Input: part model. Units: mm. Frame: model coordinates. Coordinates: 2 decimals unless noted, no trailing zeros. Order: outer loops, then holes, each group sorted by start corner. A loop starts at its lowest first (then second) coordinate and runs counter-clockwise, first axis right, second up. Notation, with made-up numbers: (-39.5, 47) -> (9.5, 47) arc R22 ccw to (9.5, 58) -> close; hole circle Ø8 at (11.5, -30.5). An arc over 180 degrees is marked (long way). Use one line per item in the form item = value. Start each with the question number.
1) Pin query (flat end, axial travel): pin 1 (1.5 mm diameter, centred on x = 8, y = 72, fed in from -Z); pin 2 (2 mm diameter, centred on x = 8, y = 112, fed in from +Z); pin 3 (2 mm diameter, centred on x = 8, y = 72, fed in from -Z). Return the tip coordinate at first contact, or that it passes through.
2) Section query B-B on y = 82. Output: boundary loops of the cut face in (x, z).
3) Ray query, line 1 along Y through (x, z) = (8, -62); line 2 along Z through (x, y) = (8, 130.75); line 3 along Y through (x, z) = (8.5, -55). Return the intervals inside material, ascending.
4) Section query A-A on z = -25. Output: boundary loops of the cut face in (x, y), then the cut area to 3 significant figures.
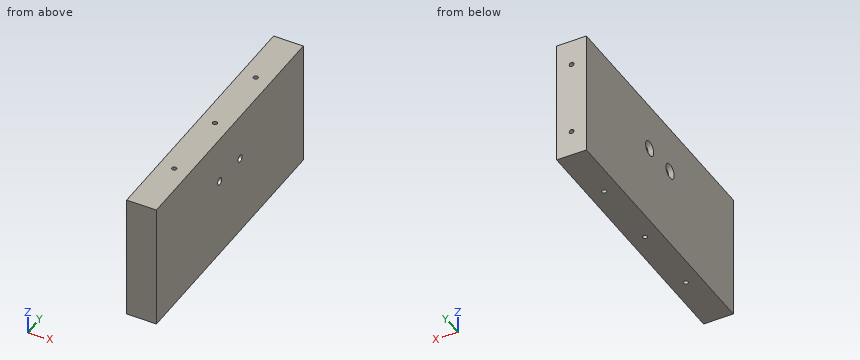
Autodesk Inventor part; units mm, degrees
ref_plane "YZ Plane" through (0, 0, 0) normal (1, 0, 0) x (0, 1, 0)
ref_plane "XZ Plane" through (0, 0, 0) normal (0, 1, 0) x (-1, 0, 0)
ref_plane "XY Plane" through (0, 0, 0) normal (0, 0, 1) x (1, 0, 0)
sketch "Skizze1" plane through (0, 0, 0) normal (1, 0, 0) x (0, 1, 0)
  line L0 (0, 0) -> (144, 0)
  line L1 (144, 0) -> (144, -68)
  line L2 (144, -68) -> (0, -68)
  line L3 (0, -68) -> (0, 0)
  dimension "d0" = 144
  dimension "d1" = 68
extrude "Extrusion1" add sketch "Skizze1" along normal blind 16
sketch "Skizze2" plane through (0, 0, 0) normal (0, 0, 1) x (1, 0, 0)
  line L0 (0, 0) -> (0, 144) construction
  line L1 (0, 72) -> (16, 72) construction
  line L2 (16, 144) -> (16, 0) construction
  line L3 (0, 144) -> (16, 144) construction
  line L4 (8, 144) -> (8, 0) construction
  line L5 (0, 144) -> (16, 144) construction
  line L6 (0, 0) -> (16, 0) construction
  line L7 (0, 144) -> (16, 144) construction
  line L8 (16, 144) -> (16, 0) construction
  line L9 (16, 0) -> (0, 0) construction
  line L10 (0, 0) -> (0, 144) construction
  line L11 (0, 112) -> (16, 112) construction
  line L12 (0, 32) -> (16, 32) construction
  point P0 (8, 112)
  point P1 (8, 72)
  point P2 (8, 32)
  dimension "d4" = 40
  dimension "d5" = 40
hole "Bohrung1" at (8, 112, 0) at (8, 72, 0) at (8, 32, 0) direction (0, 0, -1) diameter 2.5 depth 30 tip angle 118
sketch "Skizze3" plane through (0, 144, 0) normal (0, 1, 0) x (1, 0, 0)
  line L0 (0, 0) -> (16, 0)
  line L1 (16, 0) -> (16, 68)
  line L2 (16, 68) -> (0, 68)
  line L3 (0, 68) -> (0, 0)
  line L4 (8, 0) -> (8, 68) construction
  line L5 (0, 68) -> (16, 68) construction
  line L6 (16, 0) -> (16, 68) construction
  line L7 (16, 34) -> (0, 34) construction
  line L8 (0, 68) -> (0, 0) construction
  line L9 (0, 14) -> (16, 14) construction
  line L10 (0, 54) -> (16, 54) construction
  point P0 (8, 14)
  point P1 (8, 54)
  dimension "d13" = 14
  dimension "d22" = 14
hole "Bohrung2" at (8, 144, -14) at (8, 144, -54) direction (0, -1, 0) diameter 2.5 depth 25 tip angle 118
sketch "Skizze4" plane through (0, 0, -68) normal (0, 0, -1) x (-1, 0, 0)
  line L0 (0, 0) -> (-16, 0) construction
  line L1 (-16, 0) -> (-16, 144) construction
  line L2 (-16, 144) -> (0, 144) construction
  line L3 (0, 144) -> (0, 0) construction
  line L4 (-8, 0) -> (-8, 144) construction
  line L5 (-16, 144) -> (-16, 0) construction
  line L6 (-16, 72) -> (0, 72) construction
  circle A0 centre (-8, 72) radius 1.25 construction
  point P0 (-8, 112)
  point P1 (-8, 32)
  dimension "d23" = 40
  dimension "d24" = 40
hole "Bohrung3" at (8, 72, -68) at (8, 112, -68) at (8, 32, -68) direction (0, 0, 1) diameter 2.5 depth 30 tip angle 118
sketch "Skizze6" plane through (0, 0, 0) normal (-1, 0, 0) x (0, 0, 1)
  line L0 (0, 0) -> (-68, 0) construction
  line L1 (-68, 0) -> (-68, 144) construction
  line L2 (-68, 144) -> (0, 144) construction
  line L3 (0, 144) -> (0, 0) construction
  line L4 (0, 144) -> (0, 0) construction
  line L5 (0, 72) -> (-68, 72) construction
  line L6 (-68, 70.75) -> (-68, 73.25) construction
  line L7 (0, 0) -> (-68, 0) construction
  line L8 (-34, 0) -> (-34, 144) construction
  line L9 (0, 144) -> (-68, 144) construction
  line L10 (-25, 82) -> (-25, 62) construction
  point P0 (-25, 72)
  dimension "d41" = 25
  dimension "d42" = 10
hole "Bohrung5" at (0, 82, -25) at (0, 62, -25) direction (1, 0, 0) diameter 4 end through all countersink diameter 8 countersink angle 90
equation "\"d48\" = Stärke"
equation "\"Biegeradius\" = Stärke"
equation "\"BreiteBiegungsfreistellung\" = Stärke"
equation "\"TiefeBiegungsfreistellung\" = 0.5 * Stärke"
equation "\"GrößeEckenfreistellung\" = 4 * Stärke"
equation "\"MinimalRest\" = 2 * Stärke"
equation "\"Übergangsradius\" = Biegeradius"
equation "\"JacobiRadiusGröße\" = Biegeradius"
equation "\"Abstandsgröße\" = Stärke"
properties part number "licht_200_side_left" material "Spanplatte"
Answers below:
q1.pin_1 = -37.7
q1.pin_2 = -30.15
q1.pin_3 = -37.85
q2.outline = (0, -68) -> (16, -68) -> (16, -27) -> (2, -27) -> (0, -29) -> close; (0, -21) -> (2, -23) -> (16, -23) -> (16, 0) -> (0, 0) -> close
q3.line_1 = 0 to 30.75, 33.25 to 70.75, 73.25 to 110.75, 113.25 to 144
q3.line_2 = -68 to -55.25, -52.75 to -15.25, -12.75 to 0
q3.line_3 = 0 to 30.85, 33.15 to 70.85, 73.15 to 110.85, 113.15 to 118.92
q4.outline = (0, 0) -> (16, 0) -> (16, 60) -> (2, 60) -> (0, 58) -> close; (0, 66) -> (2, 64) -> (16, 64) -> (16, 80) -> (2, 80) -> (0, 78) -> close; (0, 86) -> (2, 84) -> (16, 84) -> (16, 144) -> (0, 144) -> close; hole circle Ø2.5 at (8, 32); hole circle Ø2.5 at (8, 72); hole circle Ø2.5 at (8, 112)
q4.area = 2,150 mm^2
